```python
from build123d import *

# Parameters (mm, degrees)
BASE_DEPTH                    = 10
TOWER_SKETCH_W                = 29.999999999999996
TOWER_SKETCH_H                = 30
TOWER_DEPTH                   = 70
BASE_RADIUS_R                 = 20
BASE_SCREW_D                  = 6.6
BASE_SCREW_CBORE_D            = 11
BASE_SCREW_CBORE_DEPTH        = 24
TOWER_BEVEL_SIZE              = 50
TOWER_BEVEL_SIZE_2            = 6.139228045
TOP_COVER_SCREW_HOLE_SKETCH_R = 3.950000000000002
COVER_SREW_HOLE_DEPTH         = 15
P_IDAT_VYSUNUT_M3_DEPTH       = 3
PROFILE_BEVEL_SIZE            = 3
ROUNDING_R                    = 5


# Some blends are built 0.0001 mm under size
with BuildPart() as part:
    # Base sketch → Base (new body)
    with BuildSketch(Plane.XY):
        Polygon((-30.000000000000007, 15.000000000000002), (29.999999999999986, 15.000000000000002), (29.999999999999993, -14.999999999999998), (-30, -14.999999999999998), align=None)
    extrude(amount=BASE_DEPTH)

    # Tower sketch → Tower (add)
    with BuildSketch(Plane.XY.offset(10)):
        with Locations((14.999999999999988, 1.78e-15)):
            Rectangle(TOWER_SKETCH_W, TOWER_SKETCH_H)
    extrude(amount=TOWER_DEPTH)

    # Base radius
    base_radius_edges = [part.edges().sort_by_distance(p)[0] for p in [
        (-1.041e-14, 1.78e-15, 10),
    ]]
    fillet(base_radius_edges, radius=BASE_RADIUS_R)

    # Base screw (through all)
    with Locations(Plane.XY.offset(30)):
        with Locations((-15, 0)):
            CounterBoreHole(BASE_SCREW_D / 2, BASE_SCREW_CBORE_D / 2, BASE_SCREW_CBORE_DEPTH)

    # tower bevel
    # the kernel refuses this chamfer: 50, 6.139228045 mm, written as the material it takes off along each edge
    with BuildSketch(Plane(origin=(159.96415924997035, 15.000000000000002, 80), x_dir=(0, 0.004688575069790863, -0.9999890085715016), z_dir=(-1, 0, 0))) as tower_bevel_piece_1:
        Polygon((TOWER_BEVEL_SIZE * 0.999989008572, TOWER_BEVEL_SIZE * 0.00468857506979), (-TOWER_BEVEL_SIZE_2 * 0.0046885750699, TOWER_BEVEL_SIZE_2 * 0.999989008595), (0, 0), align=None)
    extrude(amount=289.9283184999407, mode=Mode.SUBTRACT)
    with BuildSketch(Plane(origin=(-1.041e-14, 144.96415924997035, 80), x_dir=(-0.00468857506979085, 0, -0.9999890085715016), z_dir=(0, -1, 0))) as tower_bevel_piece_2:
        Polygon((TOWER_BEVEL_SIZE * 0.999989008572, TOWER_BEVEL_SIZE * 0.00468857506979), (-TOWER_BEVEL_SIZE_2 * 0.0046885750699, TOWER_BEVEL_SIZE_2 * 0.999989008595), (0, 0), align=None)
    extrude(amount=289.9283184999407, mode=Mode.SUBTRACT)
    with BuildSketch(Plane(origin=(-129.96415924997035, -14.999999999999998, 80), x_dir=(0, 0.9548873060039238, 0.2969684037613576), z_dir=(1, 0, 0))) as tower_bevel_piece_3:
        Polygon((TOWER_BEVEL_SIZE_2 * 0.954887306027, -TOWER_BEVEL_SIZE_2 * 0.296968403768), (-TOWER_BEVEL_SIZE * 0.296968403761, -TOWER_BEVEL_SIZE * 0.954887306004), (0, 0), align=None)
    extrude(amount=289.9283184999407, mode=Mode.SUBTRACT)

    # Top cover screw hole sketch → Cover srew hole (cut)
    with BuildSketch(Plane.XY.offset(80)):
        with Locations((18.06961402257261, 2.6e-15)):
            Circle(TOP_COVER_SCREW_HOLE_SKETCH_R)
    extrude(amount=-COVER_SREW_HOLE_DEPTH, mode=Mode.SUBTRACT)

    # profile sketch → Přidat vysunutím3 (add)
    with BuildSketch(Plane(origin=(0, 0, 0), x_dir=(-1, 0, 0), z_dir=(0, 0, -1))):
        with BuildLine():
            Line((8.071796769724529, 4), (-30, 4))
            Line((-30, 4), (-30, -4))
            Line((-30, -4), (8.071796769724536, -4))
            ThreePointArc((8.071796769724518, -4.000000000000045), (7.000000000000002, 9.8e-16), (8.071796769724518, 4.0000000000000435))
        make_face()
        with BuildLine():
            Line((30.000000000000007, 4), (21.928203230275386, 4))
            ThreePointArc((21.928203230275436, 4.0000000000001386), (22.72740661031253, 2.070552360820243), (23.000000000000007, 0))
            ThreePointArc((23.000000000000007, -1.96e-15), (22.72740661031253, -2.0705523608202414), (21.928203230275436, -4.000000000000134))
            Line((21.928203230275393, -4), (30.000000000000007, -4))
            Line((30.000000000000007, -4), (30.000000000000007, 4))
        make_face()
    extrude(amount=P_IDAT_VYSUNUT_M3_DEPTH)

    # Profile bevel
    profile_bevel_edges = [part.edges().sort_by_distance(p)[0] for p in [
        (-23.000000000000007, 3.22e-15, -3),
    ]]
    chamfer(profile_bevel_edges, length=PROFILE_BEVEL_SIZE - 0.0001)  # a hair under: the kernel refuses the full size

    # rounding
    rounding_edges = [part.edges().sort_by_distance(p)[0] for p in [
        (-30, -14.999999999999998, 5),
        (-30.000000000000007, 15.000000000000002, 5),
    ]]
    fillet(rounding_edges, radius=ROUNDING_R)


solid = part.part
```
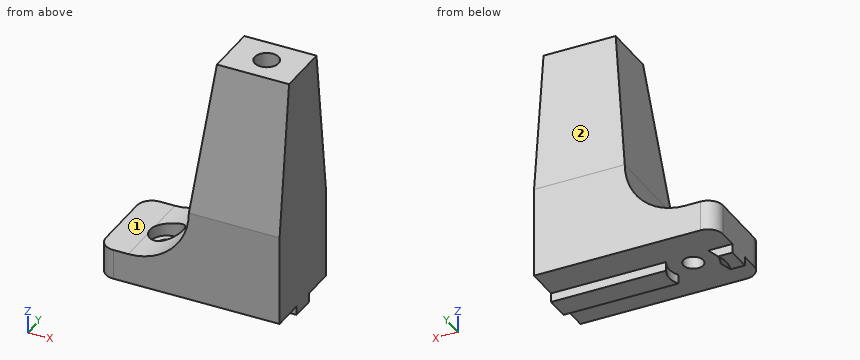
Design review of the part built by this model. Coordinates are the model's own, in mm. Face numbers are marked on the shaded views. A direction names the side the tool comes from. Give positions to 0.01 mm unless a question says otherwise; leave off trailing zeros. Write each loop counter-clockwise with the first axis right and the second up, starting at its lowest first coordinate (ties: lowest second). Pieces come first, ordered by that corner, then holes. Notation, with made-up numbers: (2.25, 37) - (20.25, 37) arc R12 cw to (20.25, 59) - close; hole circle Ø1 at (87.25, 49). An arc over 180 degrees is marked (long way). Return JSON: item names as keys, results as strings. Group by question number.
(1) We need section D-D, the plane x = 13. Give the boundary of the cut face in (y, z).
(2) Machinability: for the marked faces 1 and 2, which of the approach directions +Z, -Z, +X, -X, +Y, -Y give a long, thin tool a straight path to every point of the face, cutting with its end or side? Answer none if there is none.
(3) We need section C-C, the plane z = 67.5. Give the boundary of the cut face in (x, y).
(4) We need section B-B, the plane x = -15. Give the boundary of the cut face in (y, z), then the cut area to 3 significant figures.
(5) To check wall thickness, follow probe 1 along Z at (x, y) = (17, 6); probe 2 along X at (y, z) = (-2.5, 69); probe 3 along Z at (x, y) = (-19.5, -7). State the ranges of each line that lie inside material, in increasing order.
(6) Insertion check: pin 1 (12 mm diameter, centred on y = 9.5, z = 57, fed in from -X); pin 2 (10 mm diameter, centred on y = 2, z = 24, fed in from -X); pin 3 (10 mm diameter, centred on x = 0, y = 11, fed in from -Z). Each pin has a flat end and moves straight along its axis. Give the tip position at first contact, or say it passes through.
Reported:
{
 "1": {"outline": "(-15, 0) - (-4, 0) - (-4, -3) - (4, -3) - (4, 0) - (15, 0) - (15, 30) - (8.86, 80) - (-8.86, 80) - (-15, 30) - close"},
 "2": {"face 1": "+Z, -X, +Y, -Y", "face 2": "+Z, +X, -X, +Y"},
 "3": {"outline": "(4.6, -10.4) - (30, -10.4) - (30, 10.4) - (4.6, 10.4) - close; hole circle Ø7.9 at (18.07, 0)"},
 "4": {"outline": "(-15, 0) - (-3.3, 0) - (-3.3, 6) - (-5.5, 6) - (-5.5, 10.64) - (-15, 10.64) - close; (3.3, 0) - (15, 0) - (15, 10.64) - (5.5, 10.64) - (5.5, 6) - (3.3, 6) - close", "area": "228 mm2"},
 "5": {"probe 1": "z = 0 to 80", "probe 2": "x = 4.79 to 15.01, 21.13 to 30", "probe 3": "z = 0 to 10.01"},
 "6": {"pin 1": "stops at x = 2.58", "pin 2": "stops at x = -3.3", "pin 3": "stops at z = 0"}
}
